from build123d import *
from build123d import SkipClean  # not in build123d's __all__

# Parameters (mm, degrees)
F0_R     = 3
F0_R_2   = 1.8
F1_DEPTH = 13
F2_R     = 1.8
F3_DEPTH = 1.5
F4_W     = 6
F4_H     = 6
F5_DEPTH = 1


with BuildPart() as f1:
    # F0 (on Top) → F1 (new body)
    with BuildSketch(Plane.XY):
        with Locations((-14, 14)):
            Circle(F0_R)
        with Locations((-14, 14)):
            Circle(F0_R_2, mode=Mode.SUBTRACT)
    extrude(amount=F1_DEPTH)



with BuildPart() as f1b:
    # F0 (on Top) → F1, piece 2 (new body)
    with BuildSketch(Plane.XY):
        with Locations((-14, -14)):
            Circle(F0_R)
        with Locations((-14, -14)):
            Circle(F0_R_2, mode=Mode.SUBTRACT)
    extrude(amount=F1_DEPTH)


with BuildPart() as f1c:
    # F0 (on Top) → F1, piece 3 (new body)
    with BuildSketch(Plane.XY):
        with Locations((14, -14)):
            Circle(F0_R)
        with Locations((14, -14)):
            Circle(F0_R_2, mode=Mode.SUBTRACT)
    extrude(amount=F1_DEPTH)


with BuildPart() as f1d:
    # F0 (on Top) → F1, piece 4 (new body)
    with BuildSketch(Plane.XY):
        with Locations((14, 14)):
            Circle(F0_R)
        with Locations((14, 14)):
            Circle(F0_R_2, mode=Mode.SUBTRACT)
    extrude(amount=F1_DEPTH)


with BuildPart() as f1_1:
    add(f1.part, clean=False)

    with SkipClean():  # cleaning this boolean's faces spoils the solid; the shape is the same uncleaned
        add(f1b.part)  # F3 merges F1b

    with SkipClean():  # cleaning this boolean's faces spoils the solid; the shape is the same uncleaned
        add(f1c.part)  # F3 merges F1c

    with SkipClean():  # cleaning this boolean's faces spoils the solid; the shape is the same uncleaned
        add(f1d.part)  # F3 merges F1d
    # F2 (on face) → F3 (join)
    with BuildSketch(Plane.XY.offset(13)):
        with BuildLine():
            Line((14, 17), (-14, 17))
            ThreePointArc((-14, 17), (-16.1213203436, 16.1213203436), (-17, 14))
            Line((-17, 14), (-17, -14))
            ThreePointArc((-17, -14), (-16.1213203436, -16.1213203436), (-14, -17))
            Line((-14, -17), (14, -17))
            ThreePointArc((14, -17), (16.1213203436, -16.1213203436), (17, -14))
            Line((17, -14), (17, 14))
            ThreePointArc((17, 14), (16.1213203436, 16.1213203436), (14, 17))
        make_face()
        with Locations((-14, -14)):
            Circle(F2_R, mode=Mode.SUBTRACT)
        with Locations((14, -14)):
            Circle(F2_R, mode=Mode.SUBTRACT)
        with Locations((-14, 14)):
            Circle(F2_R, mode=Mode.SUBTRACT)
        with BuildLine():
            Line((-15, -11.1715728753), (-15, 11.1715728753))
            ThreePointArc((-15, 11.1715728753), (-11.8786796564, 11.8786796564), (-11.1715728753, 15))
            Line((-11.1715728753, 15), (11.1715728753, 15))
            ThreePointArc((11.1715728753, 15), (11.8786796564, 11.8786796564), (15, 11.1715728753))
            Line((15, 11.1715728753), (15, -11.1715728753))
            ThreePointArc((15, -11.1715728753), (11.8786796564, -11.8786796564), (11.1715728753, -15))
            Line((11.1715728753, -15), (-11.1715728753, -15))
            ThreePointArc((-11.1715728753, -15), (-11.8786796564, -11.8786796564), (-15, -11.1715728753))
        make_face(mode=Mode.SUBTRACT)
        with Locations((14, 14)):
            Circle(F2_R, mode=Mode.SUBTRACT)
    with SkipClean():  # cleaning this boolean's faces spoils the solid; the shape is the same uncleaned
        extrude(amount=F3_DEPTH)

    # F4 (on face) → F5 (join)
    with BuildSketch(Plane.XY.offset(14.5)):
        Polygon((1, 15), (-1, 15), (-1, 9), (-7, 9), (-7, 15), (-9, 15), (-9, 9), (-15, 9), (-15, 7), (-9, 7), (-9, 1), (-15, 1), (-15, -1), (-9, -1), (-9, -7), (-15, -7), (-15, -9), (-9, -9), (-9, -15), (-7, -15), (-7, -9), (-1, -9), (-1, -15), (1, -15), (1, -9), (7, -9), (7, -15), (9, -15), (9, -9), (15, -9), (15, -7), (9, -7), (9, -1), (15, -1), (15, 1), (9, 1), (9, 7), (15, 7), (15, 9), (9, 9), (9, 15), (7, 15), (7, 9), (1, 9), align=None)
        with Locations((-4, -4)):
            Rectangle(F4_W, F4_H, mode=Mode.SUBTRACT)
        with Locations((4, -4)):
            Rectangle(F4_W, F4_H, mode=Mode.SUBTRACT)
        with Locations((-4, 4)):
            Rectangle(F4_W, F4_H, mode=Mode.SUBTRACT)
        with Locations((4, 4)):
            Rectangle(F4_W, F4_H, mode=Mode.SUBTRACT)
    extrude(amount=-F5_DEPTH)


solid = f1_1.part
Part model, mm, in its own coordinate system. A direction names the side the tool comes from. Give positions to 0.01 mm unless a question says otherwise; leave off trailing zeros. Write each loop counter-clockwise with the first axis right and the second up, starting at its lowest first coordinate (ties: lowest second). Pieces come first, ordered by that corner, then holes.
1) Pin check, flat tips, straight feed: pin 1 (5 mm diameter, centred on y = 11, z = 3, fed in from +X); pin 2 (1.5 mm diameter, centred on y = 11, z = 6.5, fed in from +X); pin 3 (3 mm diameter, centred on x = -0.5, y = 2, fed in from -Z). Stop position of each tip, or through.
Resolved:
pin 1: stops at x = 16.96
pin 2: stops at x = 15.98
pin 3: stops at z = 13.5
2) Cut at B-B on z = 12.25. Write the cut outline in (x, y), then the cut area to 3 significant figures.
Resolved:
outline: circle Ø6 at (-14, -14); circle Ø6 at (-14, 14); circle Ø6 at (14, -14); circle Ø6 at (14, 14); hole circle Ø3.6 at (-14, -14); hole circle Ø3.6 at (-14, 14); hole circle Ø3.6 at (14, -14); hole circle Ø3.6 at (14, 14)
area: 72.4 mm2
3) Probe L1, parallel to Y at x = 14, z = 8.5; L2, parallel to Y at x = 14.5, z = 11; L3, parallel to X at y = -15, z = 11.75. List the from-to ranges inside material, lowest first.
Resolved:
L1: y = -17 to -15.8, -12.2 to -11, 11 to 12.2, 15.8 to 17
L2: y = -16.96 to -15.73, -12.27 to -11.04, 11.04 to 12.27, 15.73 to 16.96
L3: x = -16.83 to -15.5, -12.5 to -11.17, 11.17 to 12.5, 15.5 to 16.83
4) Which spindle directions (+Z, -Z, +X, -X, +Y, -Y) get a long thin tool onto all of the face, cutting with end or side? Do faces 1 (the face through (-12, 1, 14)), 2 (the face through (15, 0.2, 13.2)). Say none if no direction does.
Resolved:
face 1: +Z, -Z
face 2: -Z
5) Cut at A-A on x = 10. Write the cut outline in (y, z), then the cut area to 3 significant figures.
Resolved:
outline: (-17, 13) - (-15, 13) - (-15, 14.5) - (-17, 14.5) - close; (-9, 13.5) - (-7, 13.5) - (-7, 14.5) - (-9, 14.5) - close; (-1, 13.5) - (1, 13.5) - (1, 14.5) - (-1, 14.5) - close; (7, 13.5) - (9, 13.5) - (9, 14.5) - (7, 14.5) - close; (15, 13) - (17, 13) - (17, 14.5) - (15, 14.5) - close
area: 12.0 mm2
6) Two-plate mould, pull along Y, no slides. Class faces 3 (the face through (-17, 0, 14)), 4 (the face through (-4, 1, 14)): released by +Y, released by -Y, zero draft, split by the parting line, or undercut.
Resolved:
face 3: zero draft
face 4: undercut
7) Cut at D-D on y = -8. Write the cut outline in (x, z).
Resolved:
outline: (-17, 13) - (-15, 13) - (-15, 13.5) - (15, 13.5) - (15, 13) - (17, 13) - (17, 14.5) - (-17, 14.5) - close
